Design review of the part built by this model. Coordinates are the model's own, in mm. A direction names the side the tool comes from. Coordinates: 2 decimals unless noted, no trailing zeros. Order: outer loops, then holes, each group sorted by start corner. A loop starts at its lowest first (then second) coordinate and runs counter-clockwise, first axis right, second up. Notation, with made-up numbers: (18, -5) -> (34, -5) arc R18 ccw to (34, 29) -> close; hole circle Ø1 at (69, 40). An arc over 180 degrees is marked (long way). Write item = value, one per line.
```python
from build123d import *

# Parameters (mm, degrees)
SKETCH2_W           = 127
SKETCH2_H           = 76.2
BOSS_EXTRUDE1_DEPTH = 2.9718
SKETCH3_R           = 1.5875
CUT_EXTRUDE1_DEPTH  = 2.9718


with BuildPart() as part:
    # Sketch2 → Boss-Extrude1 (new body)
    with BuildSketch(Plane(origin=(0, 0, 0), x_dir=(1, 0, 0), z_dir=(0, 1, 0))):
        Rectangle(SKETCH2_W, SKETCH2_H)
    extrude(amount=BOSS_EXTRUDE1_DEPTH)

    # Sketch3 → Cut-Extrude1 (cut)
    with BuildSketch(Plane(origin=(0, 2.9718, 0), x_dir=(1, 0, 0), z_dir=(0, 1, 0))):
        Polygon((4.978749596, -4.724789245), (4.978749596, -2.54), (-38.1, -2.54), (-38.1, -38.1), (38.1, -38.1), (38.1, -9.614135395), (31.086734384, -9.614135395), (31.086734384, -4.724789245), align=None)
        with Locations((41.275, -34.925)):
            Circle(SKETCH3_R)
        with Locations((47.625, -34.925)):
            Circle(SKETCH3_R)
        with Locations((-41.275, -34.925)):
            Circle(SKETCH3_R)
        with Locations((-47.625, -34.925)):
            Circle(SKETCH3_R)
    cut_extrude1 = extrude(amount=-CUT_EXTRUDE1_DEPTH, mode=Mode.SUBTRACT)

    # Mirror1: Cut-Extrude1 across plane
    add(cut_extrude1.mirror(Plane.XY), mode=Mode.SUBTRACT)


solid = part.part
```
(1) For L1, parallel to X at y = 1.2, z = 12.5; L2, parallel to X at y = 0.7, z = 9; L3, parallel to X at y = 2.75, z = -33.5, list the stretches that pass through material, from the lowest coordinate up.
Report:
L1 = -63.5 to -38.1, 38.1 to 63.5
L2 = -63.5 to -38.1, 31.09 to 63.5
L3 = -63.5 to -48.32, -46.93 to -41.97, -40.58 to -38.1, 38.1 to 40.58, 41.97 to 46.93, 48.32 to 63.5
(2) We need section D-D (x = -19.5). Write out the cut boundary in (y, z), and give its area (3 significant figures).
Report:
outline = (0, -2.54) -> (2.97, -2.54) -> (2.97, 2.54) -> (0, 2.54) -> close
area = 15.1 mm²
(3) For faces 1 (the flat face through (18, 2, -4.725)), 2 (the cylindrical face through (49.091, 1.507, 35.533)), 3 (the flat face through (-16, 2, 2.54)), list the 3-axis set-ups (+Z, -Z, +X, -X, +Y, -Y) from which the entire face can be reached by the end or side of a thin tool; tool diameter is ignored.
Report:
face_1 = -Z, +Y, -Y
face_2 = +Y, -Y
face_3 = +Z, +Y, -Y
(4) Insertion check: pin 1 (3 mm diameter, centred on x = -47.625, z = -34.925, fed in from -Y); pin 2 (0.9 mm diameter, centred on x = 35, y = 1.5, fed in from +Z); pin 3 (0.9 mm diameter, centred on x = 34, y = 2, fed in from -Z); pin 4 (0.9 mm diameter, centred on x = -12.5, y = 1, fed in from -Z). Each pin has a flat end and moves straight along its axis. Give the tip position at first contact, or say it passes through.
Report:
pin_1 = through
pin_2 = 9.61
pin_3 = -9.61
pin_4 = -2.54
(5) We need section A-A (z = 19). Write out the cut boundary in (x, y).
Report:
outline = (-63.5, 0) -> (-38.1, 0) -> (-38.1, 2.97) -> (-63.5, 2.97) -> close; (38.1, 0) -> (63.5, 0) -> (63.5, 2.97) -> (38.1, 2.97) -> close
(6) The part is to be moulded in two halves that separate along Z. For faces 4 (the cylindrical face through (-41.619, 1.507, -36.475)), 5 (the flat face through (35, 2, 9.614)), 6 (the flat face through (31.087, 2, -7)), say which applies: released by +Z, released by -Z, zero draft, split by the parting line, or undercut.
Report:
face_4 = undercut
face_5 = released by +Z
face_6 = zero draft
(7) We need section B-B (y = 0.8). Give the number of separate pieces and of enclosed holes in the cut face, and give its area (3 significant figures).
Report:
separate_pieces = 1
enclosed_holes = 8
area = 4,410 mm²
(8) We need section C-C (x = 25). Write out the cut boundary in (y, z), and give its area (3 significant figures).
Report:
outline = (0, -4.72) -> (2.97, -4.72) -> (2.97, 4.72) -> (0, 4.72) -> close
area = 28.1 mm²
